```python
from build123d import *

# Parameters (mm, degrees)
SKETCH1_R           = 16.25
BOSS_EXTRUDE1_DEPTH = 5
SKETCH2_R           = 3.5
CUT_EXTRUDE1_DEPTH  = 2.5
SKETCH3_R           = 7.5
BOSS_EXTRUDE2_DEPTH = 40
SKETCH4_R           = 4
CUT_EXTRUDE2_DEPTH  = 46
SKETCH5_R           = 2
CUT_EXTRUDE3_DEPTH  = 43.5


with BuildPart() as part:
    # Sketch1 → Boss-Extrude1 (new body)
    with BuildSketch(Plane.XY):
        Circle(SKETCH1_R)
    extrude(amount=BOSS_EXTRUDE1_DEPTH)

    # Sketch2 → Cut-Extrude1 (cut)
    with BuildSketch(Plane.XY.offset(5)):
        with Locations((0, 12)):
            Circle(SKETCH2_R)
        with Locations((12, 0)):
            Circle(SKETCH2_R)
        with Locations((0, -12)):
            Circle(SKETCH2_R)
        with Locations((-12, 0)):
            Circle(SKETCH2_R)
    extrude(amount=-CUT_EXTRUDE1_DEPTH, mode=Mode.SUBTRACT)

    # Sketch3 → Boss-Extrude2 (add)
    with BuildSketch(Plane(origin=(0, 0, 0), x_dir=(-1, 0, 0), z_dir=(0, 0, -1))):
        Circle(SKETCH3_R)
    extrude(amount=BOSS_EXTRUDE2_DEPTH)

    # Sketch4 → Cut-Extrude2 (cut, through all)
    with BuildSketch(Plane.XY.offset(5)):
        Circle(SKETCH4_R)
    extrude(amount=-CUT_EXTRUDE2_DEPTH, mode=Mode.SUBTRACT)

    # Sketch5 → Cut-Extrude3 (cut, through all)
    with BuildSketch(Plane.XY.offset(2.5)):
        with Locations((12, 0)):
            Circle(SKETCH5_R)
        with Locations((0, -12)):
            Circle(SKETCH5_R)
        with Locations((-12, 0)):
            Circle(SKETCH5_R)
        with Locations((0, 12)):
            Circle(SKETCH5_R)
    extrude(amount=-CUT_EXTRUDE3_DEPTH, mode=Mode.SUBTRACT)


solid = part.part
```
Design review of the part built by this model. Coordinates are the model's own, in mm. A direction names the side the tool comes from. Round coordinates to 2 decimals unless told otherwise and drop trailing zeros. Write each loop counter-clockwise with the first axis right and the second up, starting at its lowest first coordinate (ties: lowest second). Pieces come first, ordered by that corner, then holes.
Item 1: We need section A-A on x = 0. Write out the cut boundary in (y, z).
Item 2: Clearance check with flat-ended pins moving along their axes: pin 1 Ø8 at (y, z) = (1.5, -32.5) entering from +X; pin 2 Ø3.5 at (x, y) = (0, 12) entering from +Z; pin 3 Ø1.5 at (y, z) = (-2, -21) entering from -X; pin 4 Ø12 at (x, z) = (-4.5, -7.5) entering from +Y. State where each tip first meets the part, or that it passes through.
Item 3: The part is to be moulded in two halves that separate along Y. For faces 4 (the cylindrical face through (15.5, 4.88, 2.46)), 5 (the cylindrical face through (-0.759, -15.417, 3.768)), 6 (the flat face through (3, -3, 5)), 7 (the flat face through (2, -14, 2.5)), say which applies: +Y half, -Y half, draft (parallel to the pull), parting line (faces both ways), or undercut.
Item 4: For probe 1 along Y at (x, z) = (0, 3.6); probe 2 along X at (y, z) = (1, -12); probe 3 along Z at (x, y) = (5, -9), list the stretches that pass through material, from the lowest coordinate up.
Item 5: We need section D-D on z = 1. Write out the cut boundary in (x, y), and give its area (3 significant figures).
Item 6: We need section C-C on x = -12. Write out the cut boundary in (y, z), and give its area (3 significant figures).
Item 7: For faces 1 (the cylindrical face through (10.4, -1.2, 1.3)), 2 (the cylindrical face through (-15.497, 0.154, 3.768)), 3 (the cylindrical face through (7.493, 0.33, -19.72)), list the 3-axis set-ups (+Z, -Z, +X, -X, +Y, -Y) from which the entire face can be reached by the end or side of a thin tool; tool diameter is ignored.
Returned:
1. outline: (-16.25, 0) - (-14, 0) - (-14, 2.5) - (-15.5, 2.5) - (-15.5, 5) - (-16.25, 5) - close; (-10, 0) - (-7.5, 0) - (-7.5, -40) - (-4, -40) - (-4, 5) - (-8.5, 5) - (-8.5, 2.5) - (-10, 2.5) - close; (4, -40) - (7.5, -40) - (7.5, 0) - (10, 0) - (10, 2.5) - (8.5, 2.5) - (8.5, 5) - (4, 5) - close; (14, 0) - (16.25, 0) - (16.25, 5) - (15.5, 5) - (15.5, 2.5) - (14, 2.5) - close
2. pin 1: stops at x = 7.5
2. pin 2: passes through
2. pin 3: stops at x = -7.4
2. pin 4: stops at y = 7.5
3. face 4: parting line
3. face 5: undercut
3. face 6: draft
3. face 7: undercut
4. probe 1: y = -16.25 to -15.5, -8.5 to -4, 4 to 8.5, 15.5 to 16.25
4. probe 2: x = -7.43 to -3.87, 3.87 to 7.43
4. probe 3: z = 0 to 5
5. outline: circle Ø32.5 at (0, 0); hole circle Ø4 at (-12, 0); hole circle Ø8 at (0, 0); hole circle Ø4 at (0, -12); hole circle Ø4 at (0, 12); hole circle Ø4 at (12, 0)
5. area: 729 mm2
6. outline: (-10.96, 0) - (-2, 0) - (-2, 2.5) - (-3.5, 2.5) - (-3.5, 5) - (-10.96, 5) - close; (2, 0) - (10.96, 0) - (10.96, 5) - (3.5, 5) - (3.5, 2.5) - (2, 2.5) - close
6. area: 82.1 mm2
7. face 1: +Z, -Z
7. face 2: +Z
7. face 3: -Z
